The figure shows three views and two pictorial views of one solid part (mm, origin at its lowest corner). Answer the questions. A direction names the side the tool comes from. Give positions to 0.01 mm unless a question says otherwise; leave off trailing zeros. Loops run counter-clockwise (first coordinate to the right, second up) from the corner with the lowest first, then second, coordinate; pieces in that order, holes last.
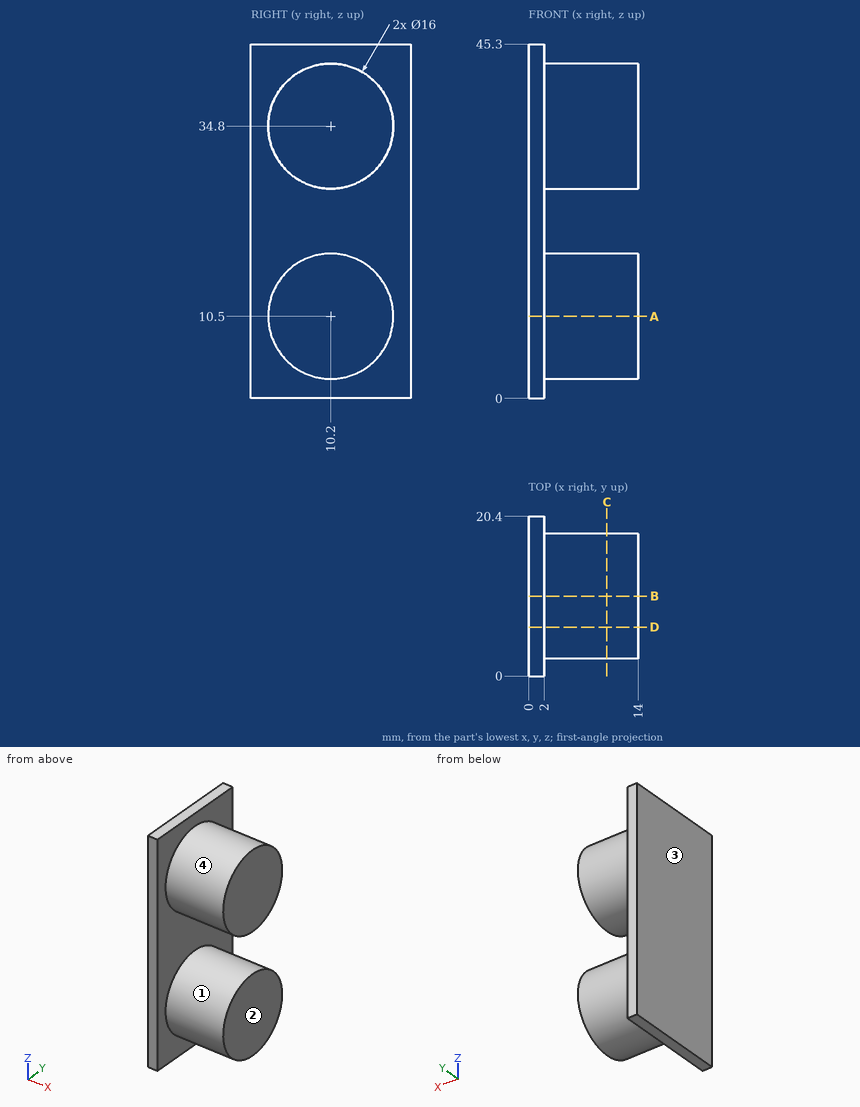
Q1. Determine the mould class of the marked faces 3 and 4 for opening direction Z: +Z half, -Z half, draft (parallel to the pull), parting line (faces both ways), or undercut.
Q2. Consider line 1 along Z through (x, y) = (5.25, 13.5); line 2 along Z through (x, y) = (11, 12.75); line 3 along X through (y, z) = (17.75, 18.5). Determine where each line is inside the solid, lowest interval first.
Q3. Section B-B on y = 10.2 is taken. Give the vertices of the cut face in (x, z).
Q4. Given pin 1 (5 mm diameter, centred on x = 11, z = 36, fed in from -Y); pin 2 (2 mm diameter, centred on x = 4.5, z = 31.5, fed in from -Y); pin 3 (1 mm diameter, centred on y = 17, z = 26.5, fed in from +X), each flat-ended and moving along its own axis, determine where each tip first touches the part or whether it passes through.
Q5. Section D-D on y = 6.25 is taken. Give the vertices of the cut face in (x, z).
Q6. Which of the six approach directions +Z, -Z, +X, -X, +Y, -Y give full straight-line access (tool end or side, diameter ignored) to the marked faces 1 and 2?
Q7. Section A-A on z = 10.5 is taken. Give the vertices of the cut face in (x, y), plus the area to 3 significant figures.
Q8. Section C-C on x = 10 is taken. Give the vertices of the cut face in (y, z), plus the area to 3 significant figures.
Check result:
1. face 3: draft
1. face 4: undercut
2. line 1: z = 3.21 to 17.79, 27.51 to 42.09
2. line 2: z = 2.92 to 18.08, 27.22 to 42.38
2. line 3: x = 0 to 2
3. outline: (0, 0) - (2, 0) - (2, 2.5) - (14, 2.5) - (14, 18.5) - (2, 18.5) - (2, 26.8) - (14, 26.8) - (14, 42.8) - (2, 42.8) - (2, 45.3) - (0, 45.3) - close
4. pin 1: stops at y = 2.2
4. pin 2: stops at y = 2.54
4. pin 3: stops at x = 2
5. outline: (0, 0) - (2, 0) - (2, 3.54) - (14, 3.54) - (14, 17.46) - (2, 17.46) - (2, 27.84) - (14, 27.84) - (14, 41.76) - (2, 41.76) - (2, 45.3) - (0, 45.3) - close
6. face 1: +X
6. face 2: +Z, -Z, +X, +Y, -Y
7. outline: (0, 0) - (2, 0) - (2, 2.2) - (14, 2.2) - (14, 18.2) - (2, 18.2) - (2, 20.4) - (0, 20.4) - close
7. area: 233 mm2
8. outline: circle Ø16 at (10.2, 10.5); circle Ø16 at (10.2, 34.8)
8. area: 402 mm2
